Could you check a few things on this drawing? It's one solid part, dimensions in mm from its lowest x, y, z. Give positions to 0.01 mm unless a question says otherwise; leave off trailing zeros. Order: outer loops, then holes, each group sorted by start corner. A loop starts at its lowest first (then second) coordinate and runs counter-clockwise, first axis right, second up.
(1) If I drill on probe 1 along Z at (x, y) = (37.5, 2.75); probe 2 along Z at (x, y) = (15, 5); probe 3 along X at (y, z) = (2.5, 5), over which ranges is the centre line in solid material (lowest first)?
(2) Will this pin go through, and if not, where does the flat tip stop? pin 1 (1.5 mm diameter, centred on x = 12.5, y = 2, fed in from -Z).
(3) Imagine slicing it at A-A, the plane x = 28. Write out the boundary of the cut face in (y, z), then the cut area to 3 significant figures.
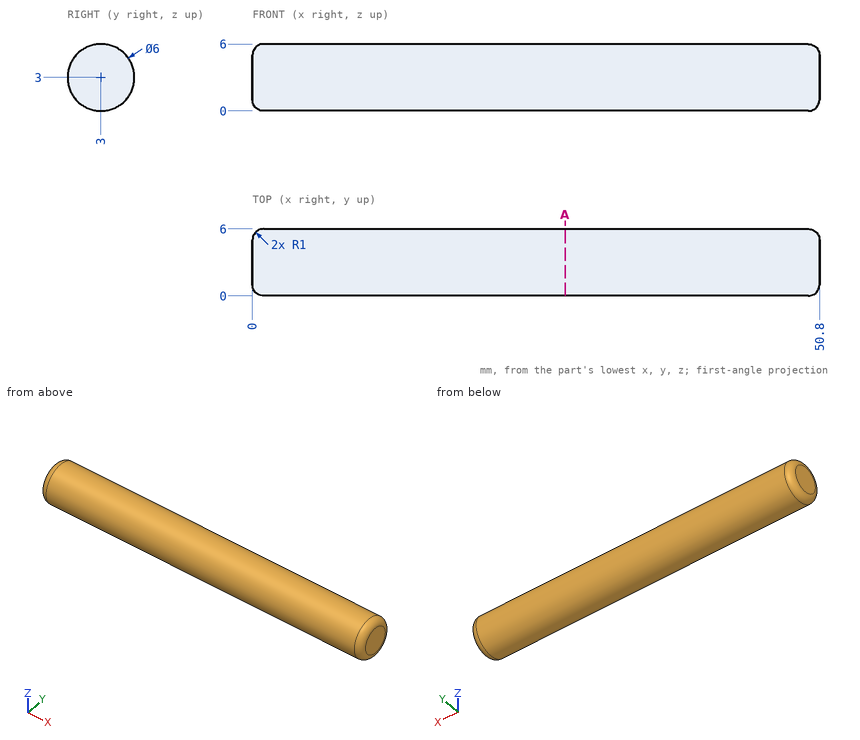
Answer block:
1. probe 1: z = 0.01 to 5.99
1. probe 2: z = 0.76 to 5.24
1. probe 3: x = 0 to 50.8
2. pin 1: stops at z = 0.01
3. outline: circle Ø6 at (3, 3)
3. area: 28.3 mm2
